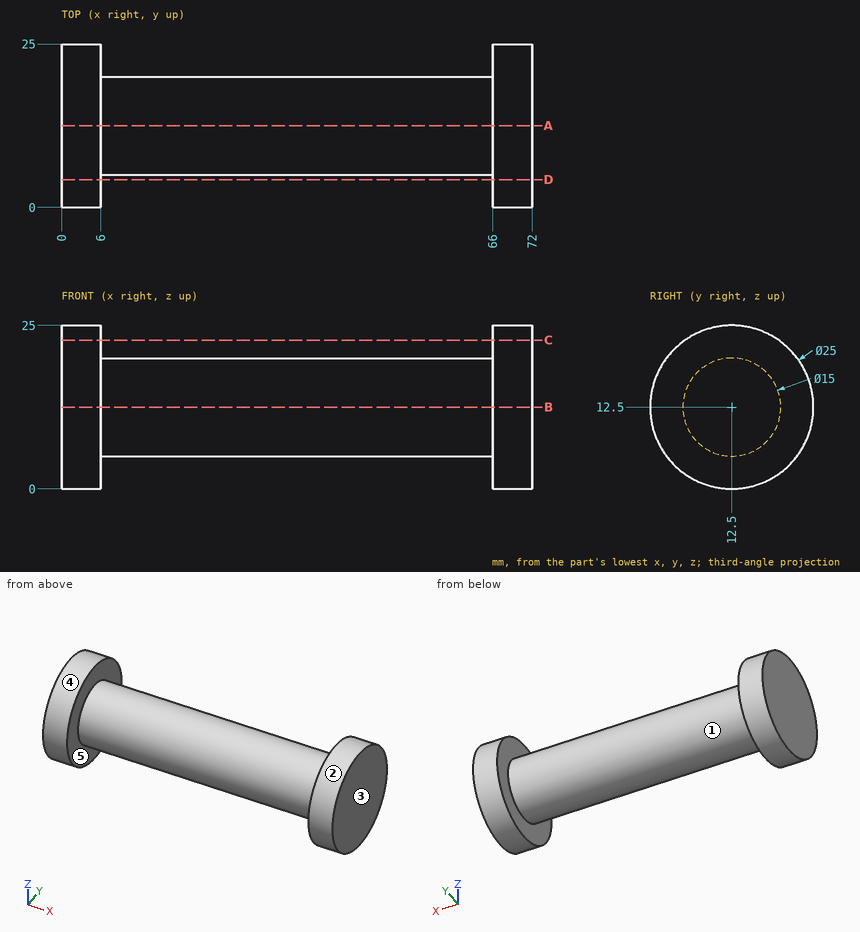
Design review of the part shown in the three views and the two pictorial views. Dimensions are in mm from the part's minimum x, y and z. A direction names the side the tool comes from. Give positions to 0.01 mm unless a question says otherwise; leave off trailing zeros. Write each loop counter-clockwise with the first axis right and the second up, starting at its lowest first coordinate (ties: lowest second). Pieces come first, ordered by that corner, then holes. Notation, with made-up numbers: (45.25, 65) - (86.25, 65) arc R26 ccw to (86.25, 89) - close; hole circle Ø10 at (6.5, -12.75). An arc over 180 degrees is marked (long way). Return JSON: item names as keys, results as strings. Group by question number.
(1) Insertion check: pin 1 (1.5 mm diameter, centred on x = 45, z = 11, fed in from -Y); pin 2 (2 mm diameter, centred on x = 52, y = 18, fed in from -Z); pin 3 (3 mm diameter, centred on x = 64, z = 19, fed in from -Y). Each pin has a flat end and moves straight along its axis. Give the tip position at first contact, or say it passes through.
(2) We need section D-D, the plane y = 4.25. Give the boundary of the cut face in (x, z), then the cut area to 3 significant figures.
(3) Mouldability with a two-part tool opening along X and no side actions: class the marked faces 1, 2 and 3 as +X half, -X half, draft (parallel to the pull), parting line (faces both ways), or undercut.
(4) We need section C-C, the plane z = 22.75. Give the boundary of the cut face in (x, y).
(5) We need section A-A, the plane y = 12.5. Give the boundary of the cut face in (x, z).
(6) Machinability: for the marked faces 4 and 5, which of the approach directions +Z, -Z, +X, -X, +Y, -Y give a long, thin tool a straight path to every point of the face, cutting with its end or side? Answer none if there is none.
(7) To check wall thickness, follow probe 1 along X at (y, z) = (7.5, 3.75); probe 2 along Z at (x, y) = (32, 12.25). State the ranges of each line that lie inside material, in increasing order.
Reported:
{
 "1": {"pin 1": "stops at y = 5.04", "pin 2": "stops at z = 6.5", "pin 3": "stops at y = 6.91"},
 "2": {"outline": "(0, 3.11) - (6, 3.11) - (6, 21.89) - (0, 21.89) - close; (66, 3.11) - (72, 3.11) - (72, 21.89) - (66, 21.89) - close", "area": "225 mm2"},
 "3": {"face 1": "undercut", "face 2": "draft", "face 3": "+X half"},
 "4": {"outline": "(0, 5.35) - (6, 5.35) - (6, 19.65) - (0, 19.65) - close; (66, 5.35) - (72, 5.35) - (72, 19.65) - (66, 19.65) - close"},
 "5": {"outline": "(0, 0) - (6, 0) - (6, 5) - (66, 5) - (66, 0) - (72, 0) - (72, 25) - (66, 25) - (66, 20) - (6, 20) - (6, 25) - (0, 25) - close"},
 "6": {"face 4": "+X, -X", "face 5": "none"},
 "7": {"probe 1": "x = 0 to 6, 66 to 72", "probe 2": "z = 5 to 20"}
}
